Geometry check sheet. Reference: the model listing, model coordinates, mm. Face numbers are marked on the shaded views. Coordinates: 2 decimals unless noted, no trailing zeros. Loops run counter-clockwise (first coordinate to the right, second up) from the corner with the lowest first, then second, coordinate; pieces in that order, holes last.
from build123d import *

# Parameters (mm, degrees)
SKETCH1_R           = 49.2125
SKETCH1_R_2         = 42.8625
BOSS_EXTRUDE1_DEPTH = 3.571875
HOLE2_D             = 3.175
HOLE2_DEPTH         = 2.38125
HOLE1_D             = 3.175
HOLE1_DEPTH         = 12.7
HOLE1_CBORE_D       = 6.35
HOLE1_CBORE_DEPTH   = 3.175
CIRPATTERN1_COUNT   = 2


with BuildPart() as part:
    # Sketch1 → Boss-Extrude1 (new body, symmetric)
    with BuildSketch(Plane(origin=(0, 0, 0), x_dir=(1, 0, 0), z_dir=(0, 1, 0))):
        Circle(SKETCH1_R)
        Circle(SKETCH1_R_2, mode=Mode.SUBTRACT)
    extrude(amount=BOSS_EXTRUDE1_DEPTH, both=True)

    # Hole2
    with Locations(Plane(origin=(49.2125, 0, 0), x_dir=(0, 0, 1), z_dir=(1, 0, 0))):
        with Locations((0, 0)):
            hole2 = Hole(HOLE2_D / 2, depth=HOLE2_DEPTH)

    # Sketch7 → #4-40 Tapped Hole1 (revolve, cut)
    with BuildSketch(Plane(origin=(46.83125, 0, 0), x_dir=(0, 0, -1), z_dir=(0, 1, 0))):
        Polygon((0, 0), (0, 9.569152758), (1.1303, 8.89), (1.1303, 0), align=None)
    f_4_40_tapped_hole1 = revolve(axis=Axis((53.18125, 0, 0), (-1, 0, 0)), mode=Mode.SUBTRACT)

    # Hole1
    with Locations(Plane(origin=(0, 0, -49.2125), x_dir=(-1, 0, 0), z_dir=(0, 0, -1))):
        with Locations((0, 0)):
            hole1 = CounterBoreHole(HOLE1_D / 2, HOLE1_CBORE_D / 2, HOLE1_CBORE_DEPTH, depth=HOLE1_DEPTH)

    # CirPattern1: Hole2, #4-40 Tapped Hole1, Hole1 ×2 about axis
    cirpattern1_axis = Axis((0, 0, 0), (0, 1, 0))
    for i in range(1, CIRPATTERN1_COUNT):
        add(hole2.rotate(cirpattern1_axis, i * 360 / CIRPATTERN1_COUNT), mode=Mode.SUBTRACT)
        add(f_4_40_tapped_hole1.rotate(cirpattern1_axis, i * 360 / CIRPATTERN1_COUNT), mode=Mode.SUBTRACT)
        add(hole1.rotate(cirpattern1_axis, i * 360 / CIRPATTERN1_COUNT), mode=Mode.SUBTRACT)


solid = part.part
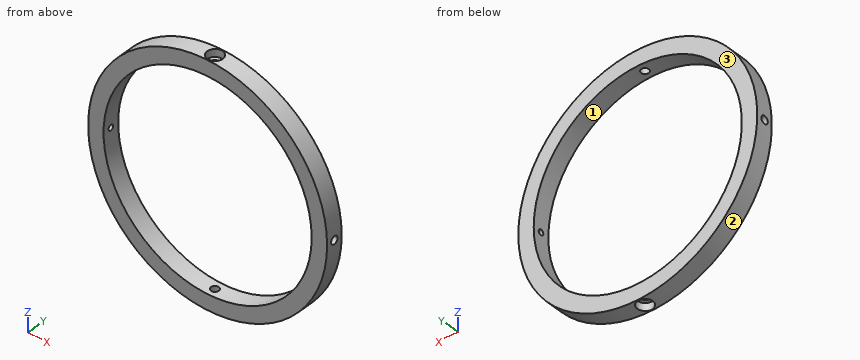
(1) Scan lines: L1, parallel to Y at x = 44, z = 0; L2, parallel to Y at x = 0, z = -48.5 (3 decimals); L3, parallel to Z at x = 12.5, y = 2.5. Record each from-to range of solid material in increasing order.
Findings:
L1: y = -3.57 to -1.13, 1.13 to 3.57
L2: y = -3.572 to -3.175, 3.175 to 3.572
L3: z = -47.6 to -41, 41 to 47.6
(2) Sectioned sample at C-C on z = -21. Record the cut outline in (x, y).
Findings:
outline: (-44.51, -3.57) - (-37.37, -3.57) - (-37.37, 3.57) - (-44.51, 3.57) - close; (37.37, -3.57) - (44.51, -3.57) - (44.51, 3.57) - (37.37, 3.57) - close
(3) Sectioned sample at B-B on x = 0. State how many separate pieces and enclosed holes the cut face has, and give its area (3 significant figures).
Findings:
separate pieces: 4
enclosed holes: 0
area: 30.2 mm2
(4) Sectioned sample at A-A on z = 0. Record the cut outline in (x, y), and give its area (3 significant figures).
Findings:
outline: (-49.21, -3.57) - (-42.86, -3.57) - (-42.86, -1.13) - (-46.83, -1.13) - (-46.83, -1.59) - (-49.21, -1.59) - close; (-49.21, 1.59) - (-46.83, 1.59) - (-46.83, 1.13) - (-42.86, 1.13) - (-42.86, 3.57) - (-49.21, 3.57) - close; (42.86, -3.57) - (49.21, -3.57) - (49.21, -1.59) - (46.83, -1.59) - (46.83, -1.13) - (42.86, -1.13) - close; (42.86, 1.13) - (46.83, 1.13) - (46.83, 1.59) - (49.21, 1.59) - (49.21, 3.57) - (42.86, 3.57) - close
area: 57.7 mm2
(5) Sectioned sample at D-D on x = 10.5. Record the cut outline in (y, z), and give its area (3 significant figures).
Findings:
outline: (-3.57, -48.08) - (3.57, -48.08) - (3.57, -41.56) - (-3.57, -41.56) - close; (-3.57, 41.56) - (3.57, 41.56) - (3.57, 48.08) - (-3.57, 48.08) - close
area: 93.2 mm2
(6) Draft check along X on the marked faces 1, 2 and 3. Enter one of: +X half, -X half, draft (parallel to the pull), parting line (faces both ways), or undercut.
Findings:
face 1: undercut
face 2: parting line
face 3: draft
(7) Gauge pin test, flat ends, axial feed: pin 1 Ø2.5 at (y, z) = (0.5, 0.5) entering from +X; pin 2 Ø2.5 at (x, y) = (0, 0) entering from +Z; pin 3 Ø3 at (x, y) = (-37, 0) entering from -Z; pin 4 Ø1.9 at (x, y) = (1.5, -0.5) entering from -Z. Record the tip position at first contact, or that the pin passes through.
Findings:
pin 1: stops at x = 49.21
pin 2: passes through
pin 3: stops at z = -34.08
pin 4: stops at z = -46.04
